Drawing for the job (mm, zero at the part's lowest x, y, z). Round coordinates to 2 decimals unless told otherwise and drop trailing zeros. Loops run counter-clockwise (first coordinate to the right, second up) from the corner with the lowest first, then second, coordinate; pieces in that order, holes last. Notation, with made-up numbers: M 87.5,-0.75 L 110.5,-0.75 A21 ccw 110.5,13.25 Z; hole C -8,34 d8. An arc over 180 degrees is marked long. Answer in a Markdown table with one row per item.
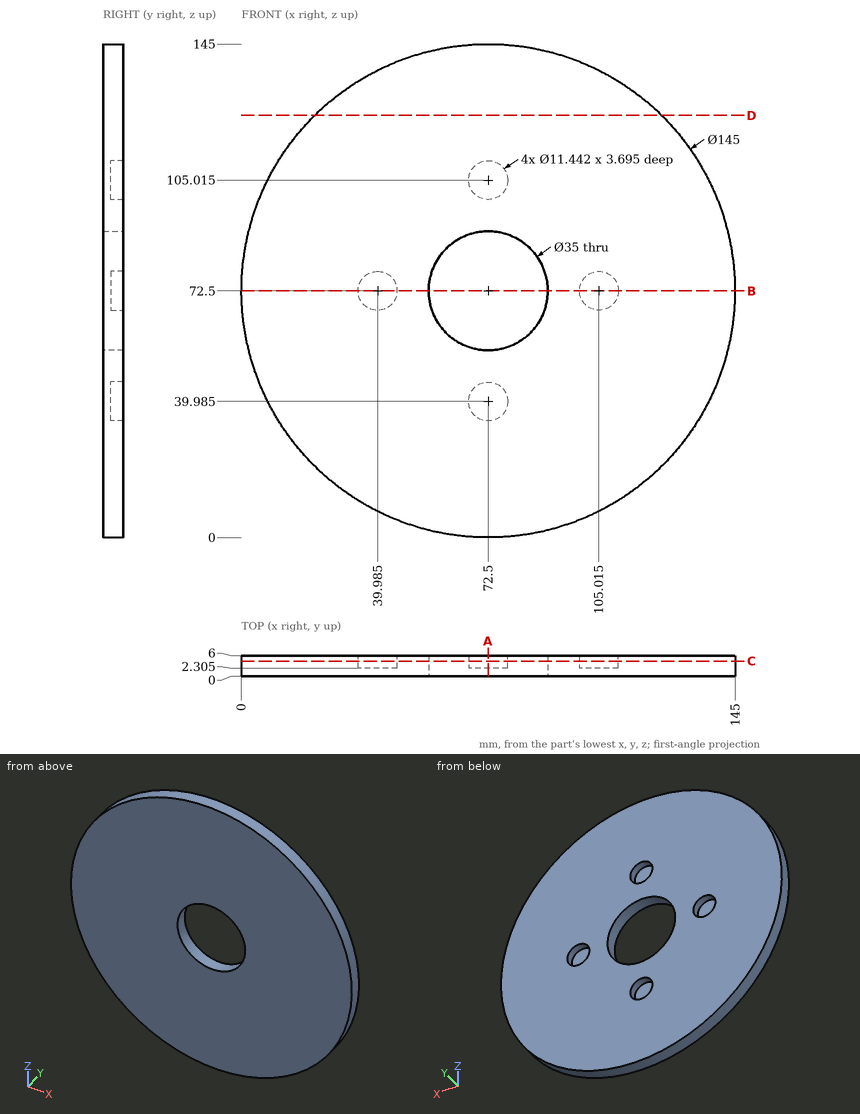
1. Saw through at B-B (z = 72.5). Write the cut outline in (x, y) (1 decimal).
Verdict:
| item | result |
|---|---|
| outline | M 0,0 L 55,0 L 55,6 L 45.7,6 L 45.7,2.3 L 34.3,2.3 L 34.3,6 L 0,6 Z; M 90,0 L 145,0 L 145,6 L 110.7,6 L 110.7,2.3 L 99.3,2.3 L 99.3,6 L 90,6 Z |
2. Saw through at A-A (x = 72.5). Write the cut outline in (y, z) (1 decimal).
Verdict:
| item | result |
|---|---|
| outline | M 0,0 L 6,0 L 6,34.3 L 2.3,34.3 L 2.3,45.7 L 6,45.7 L 6,55 L 0,55 Z; M 0,90 L 6,90 L 6,99.3 L 2.3,99.3 L 2.3,110.7 L 6,110.7 L 6,145 L 0,145 Z |
3. Pin check, flat tips, straight feed: pin 1 (1 mm diameter, centred on x = 44, z = 17.5, fed in from -Y); pin 2 (1.5 mm diameter, centred on y = 4, z = 23, fed in from +X); pin 3 (9 mm diameter, centred on x = 105.5, z = 72.5, fed in from +Y) (1 decimal); pin 4 (1 mm diameter, centred on y = 3.5, z = 60, fed in from +X). Stop position of each tip, or through.
Verdict:
| item | result |
|---|---|
| pin 1 | stops at y = 0 |
| pin 2 | stops at x = 126.16 |
| pin 3 | stops at y = 2.3 |
| pin 4 | stops at x = 144 |
4. Wall check: probe 1 along X at (y, z) = (4, 72.5); probe 2 along Y at (x, z) = (100.5, 73.5) (1 decimal); probe 3 along Z at (x, y) = (58.5, 5.3) (1 decimal). Give the ranges that are in metal, low to high.
Verdict:
| item | result |
|---|---|
| probe 1 | x = 0 to 34.26, 45.71 to 55, 90 to 99.29, 110.74 to 145 |
| probe 2 | y = 0 to 2.3 |
| probe 3 | z = 1.4 to 62, 83 to 143.6 |
5. Saw through at D-D (z = 124). Write the cut outline in (x, y).
Verdict:
| item | result |
|---|---|
| outline | M 21.47,0 L 123.53,0 L 123.53,6 L 21.47,6 Z |
6. Saw through at C-C (y = 4.35). Write the cut outline in (x, z) (1 decimal).
Verdict:
| item | result |
|---|---|
| outline | C 72.5,72.5 d145; hole C 40,72.5 d11.4; hole C 72.5,72.5 d35; hole C 72.5,40 d11.4; hole C 72.5,105 d11.4; hole C 105,72.5 d11.4 |
